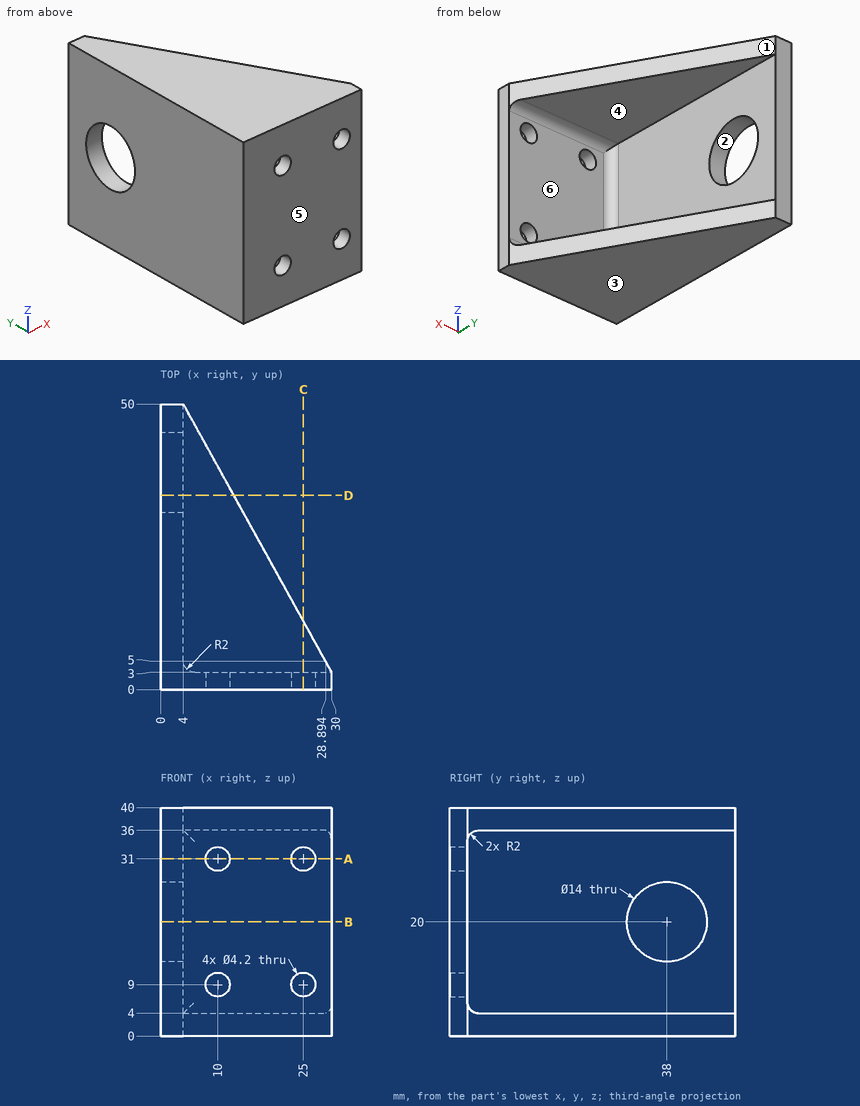
Source: three-view drawing plus pictorial views. Frame: mm from the lowest corner of the part. A direction names the side the tool comes from. Coordinates: 2 decimals unless noted, no trailing zeros. Order: outer loops, then holes, each group sorted by start corner. A loop starts at its lowest first (then second) coordinate and runs counter-clockwise, first axis right, second up.
1) Draft query along Z for the marked faces 1, 2, 3 and 4. Return one class per face: released by +Z, released by -Z, zero draft, split by the parting line, or undercut.
Result sheet:
face 1: zero draft
face 2: undercut
face 3: released by -Z
face 4: undercut
2) Section C-C (x = 25). Return loops of the section in (y, z), then the cut area to 3 significant figures.
Result sheet:
outline: (0, 0) - (12.04, 0) - (12.04, 4) - (5, 4) arc R2 cw to (3, 6) - (3, 6.9) - (0, 6.9) - close; (0, 11.1) - (3, 11.1) - (3, 28.9) - (0, 28.9) - close; (0, 33.1) - (3, 33.1) - (3, 34) arc R2 cw to (5, 36) - (12.04, 36) - (12.04, 40) - (0, 40) - close
area: 169 mm2
3) Set-up query: the marked faces 5 and 6. Return all of +Z, -Z, +X, -X, +Y, -Y with unobstructed straight access to the full face (end or side cutting, diameter ignored); none if empty.
Result sheet:
face 5: +Z, -Z, +X, -X, -Y
face 6: +X, +Y
4) Section D-D (y = 34). Return loops of the section in (x, z) (1 decimal).
Result sheet:
outline: (0, 0) - (12.9, 0) - (12.9, 4) - (4, 4) - (4, 14.3) - (0, 14.3) - close; (0, 25.7) - (4, 25.7) - (4, 36) - (12.9, 36) - (12.9, 40) - (0, 40) - close
5) Section A-A (z = 31). Return loops of the section in (x, y).
Result sheet:
outline: (0, 0) - (7.9, 0) - (7.9, 3) - (6, 3) arc R2 cw to (4, 5) - (4, 50) - (0, 50) - close; (12.1, 0) - (22.9, 0) - (22.9, 3) - (12.1, 3) - close; (27.1, 0) - (30, 0) - (30, 3) - (27.1, 3) - close
6) First-contact query: P1, Ø5.5, axis at x = 25, z = 9, coming from the +Y side; P2, Ø4, axis at x = 10, z = 9, coming from the +Y side; P3, Ø12, axis at x = 15, z = 34.5, coming from the +Y side (1 decimal); P4, Ø3, axis at y = 30.5, z = 8, coming from the +X side. Flat tips, straight axial feed; report the tip coordinate or a pass-through.
Result sheet:
P1: stops at y = 3
P2: passes through
P3: stops at y = 40.6
P4: stops at x = 4
7) Ray query, probe 1 along X at (y, z) = (2, 31); probe 2 along Z at (x, y) = (20.75, 6.5); probe 3 along Y at (x, z) = (19.75, 8.5). Return the intervals inside material, ascending.
Result sheet:
probe 1: x = 0 to 7.9, 12.1 to 22.9, 27.1 to 30
probe 2: z = 0 to 4, 36 to 40
probe 3: y = 0 to 3
8) Section B-B (z = 20). Return loops of the section in (x, y), then the cut area to 3 significant figures.
Result sheet:
outline: (0, 0) - (30, 0) - (30, 3) - (6, 3) arc R2 cw to (4, 5) - (4, 31) - (0, 31) - close; (0, 45) - (4, 45) - (4, 50) - (0, 50) - close
area: 223 mm2
